Here's how the part is built. I have some questions about the finished solid (model axes, mm). A direction names the side the tool comes from. Round coordinates to 2 decimals unless told otherwise and drop trailing zeros. Write each loop counter-clockwise with the first axis right and the second up, starting at its lowest first coordinate (ties: lowest second). Pieces come first, ordered by that corner, then holes. Notation, with made-up numbers: (-20, -33.5) -> (-6, -33.5) arc R28 ccw to (-6, -5.5) -> close; hole circle Ø2 at (-31.75, 19). An arc over 180 degrees is marked (long way). Answer as CSV lines item,"result".
from build123d import *

# Parameters (mm, degrees)
F0_R     = 10.16
F1_DEPTH = 25.4


with BuildPart() as f1:
    # F0 (on Top) → F1 (new body)
    with BuildSketch(Plane.XY):
        with Locations((-45.72, 0)):
            Circle(F0_R)
        with BuildLine():
            ThreePointArc((55.88, 0), (45.72, 10.16), (35.56, 0))
            ThreePointArc((35.56, 0), (45.72, -10.16), (55.88, 0))
        make_face()
        Polygon((-31.35884, 15.172625), (-52.64404, 15.172625), (-68.4403, -12.807356), (-30.3403, -12.807356), (-30.3403, -24.1808), (31.3563, -24.1808), (31.358133, -12.807356), (52.643333, -12.807356), (68.4403, 15.173876), (30.3403, 15.173876), (30.3403, 24.1808), (-31.35884, 24.1808), align=None)
        with Locations((-45.72, 0)):
            Circle(F0_R, mode=Mode.SUBTRACT)
        with BuildLine():
            ThreePointArc((-11.0109, 0), (0, 11.0109), (11.0109, 0))
            ThreePointArc((11.0109, 0), (0, -11.0109), (-11.0109, 0))
        make_face(mode=Mode.SUBTRACT)
        with BuildLine():
            ThreePointArc((55.88, 0), (45.72, -10.16), (35.56, 0))
            ThreePointArc((35.56, 0), (45.72, 10.16), (55.88, 0))
        make_face(mode=Mode.SUBTRACT)
    extrude(amount=F1_DEPTH)


solid = f1.part
Item 1: Suppose I cut it at A-A, the plane x = -45.72. List the corners of the cut face in (y, z) for me.
Results found:
outline,"(-12.81, 0) -> (-10.16, 0) -> (-10.16, 25.4) -> (-12.81, 25.4) -> close; (10.16, 0) -> (15.17, 0) -> (15.17, 25.4) -> (10.16, 25.4) -> close"
Item 2: Suppose I cut it at C-C, the plane y = 0. List the corners of the cut face in (x, z) for me, then the cut area to 3 significant figures.
Results found:
outline,"(-61.21, 0) -> (-55.88, 0) -> (-55.88, 25.4) -> (-61.21, 25.4) -> close; (-35.56, 0) -> (-11.01, 0) -> (-11.01, 25.4) -> (-35.56, 25.4) -> close; (11.01, 0) -> (35.56, 0) -> (35.56, 25.4) -> (11.01, 25.4) -> close; (55.88, 0) -> (59.87, 0) -> (59.87, 25.4) -> (55.88, 25.4) -> close"
area,"1,480 mm²"
Item 3: For faces 5 (the cylindrical face through (-53.783, -6.182, 12.522)), 6 (the flat face through (-30.34, -18, 13)), 7 (the flat face through (42, -12.807, 13)), 8 (the flat face through (50, 15.174, 13)), which set-ups out of +Z, -Z, +X, -X, +Y, -Y let a thin tool reach every point of the face, with its end or its side?
Results found:
face 5,"+Z, -Z"
face 6,"+Z, -Z, -X, -Y"
face 7,"+Z, -Z, +X, -Y"
face 8,"+Z, -Z, +X, +Y"
Item 4: Will these pins go through, and if not, where does the flat tip stop? pin 1 (18.5 mm diameter, centred on x = 45.72, y = 0, fed in from -Z); pin 2 (2.5 mm diameter, centred on y = 21, z = 15.5, fed in from +X); pin 3 (2 mm diameter, centred on y = 0.5, z = 6, fed in from -X); pin 4 (3 mm diameter, centred on y = 16, z = 14.5, fed in from +X).
Results found:
pin 1,"passes through"
pin 2,"stops at x = 30.34"
pin 3,"stops at x = -61.49"
pin 4,"stops at x = 68.44"
Item 5: Suppose I cut it at D-D, the plane x = 0. List the corners of the cut face in (y, z) for me, then the cut area to 3 significant figures.
Results found:
outline,"(-24.18, 0) -> (-11.01, 0) -> (-11.01, 25.4) -> (-24.18, 25.4) -> close; (11.01, 0) -> (24.18, 0) -> (24.18, 25.4) -> (11.01, 25.4) -> close"
area,"669 mm²"
Item 6: Suppose I cut it at B-B, the plane z = 22. List the corners of the cut face in (x, y) for me.
Results found:
outline,"(-68.44, -12.81) -> (-30.34, -12.81) -> (-30.34, -24.18) -> (31.36, -24.18) -> (31.36, -12.81) -> (52.64, -12.81) -> (68.44, 15.17) -> (30.34, 15.17) -> (30.34, 24.18) -> (-31.36, 24.18) -> (-31.36, 15.17) -> (-52.64, 15.17) -> close; hole circle Ø20.32 at (-45.72, 0); hole circle Ø22.02 at (0, 0); hole circle Ø20.32 at (45.72, 0)"
Item 7: I need wall thicknesses on L1, parallel to Y at x = -45.72, z = 20; L2, parallel to X at y = -3.5, z = 23.5; L3, parallel to Y at x = 0, z = 5.5. Which ranges of each line are inside material? Lowest first, please.
Results found:
L1,"y = -12.81 to -10.16, 10.16 to 15.17"
L2,"x = -63.19 to -55.26, -36.18 to -10.44, 10.44 to 36.18, 55.26 to 57.9"
L3,"y = -24.18 to -11.01, 11.01 to 24.18"
Item 8: If we mould it in two halves opening along Y, with no side actions, what happens to faces 1 (the cylindrical face through (53.783, -6.182, 12.522)), 2 (the flat face through (-31.359, 20, 13)), 3 (the flat face through (-50, -12.807, 13)), 4 (the flat face through (-42, 15.173, 13))? For each: pulls with the +Y half, pulls with the -Y half, needs draft (parallel to the pull), parting line crosses it, or undercut.
Results found:
face 1,"undercut"
face 2,"needs draft"
face 3,"pulls with the -Y half"
face 4,"pulls with the +Y half"
